Source: CAD feature listing. Evaluate the final solid. Frame: model axes, mm. A direction names the side the tool comes from. Give positions to 0.01 mm unless a question says otherwise; leave off trailing zeros. Order: outer loops, then holes, each group sorted by start corner. A loop starts at its lowest first (then second) coordinate and runs counter-clockwise, first axis right, second up. Notation, with made-up numbers: M -10.5,29.25 L 8.5,29.25 A34 cw 8.5,63.25 Z; hole C -18.5,57.25 d6. An arc over 180 degrees is marked long. Answer as a JSON object with one key per item and string values. Group by question number.
1. Section query B-B (x = 82.45). Output: boundary loops of the cut face in (y, z) (3 decimals).
2. Material intervals for L1, parallel to Z at x = 72.5, y = 22 (3 decimals); L2, parallel to X at y = 53.5, z = 9 (3 decimals); L3, parallel to Z at x = 82.45, y = -2.45 (3 decimals), sorted ascending. Write a range as [from, to].
3. Pull-direction query (X, two-part tool) for faces 1 (the flat face through (143, 11.088, 20)), 2 (the cylindrical face through (135.39, -2.15, 11.51)), 3 (the flat face through (111.252, 40, 102)); classes: +X half, -X half, draft (parallel to the pull), parting line (faces both ways), or undercut.
4. Set-up query: faces 4 (the flat face through (108, 35.1, 92)), 5 (the flat face through (143, 14.753, 52)), 6 (the flat face through (42, 15.306, -3)), 7 (the flat face through (121.69, 32, 69)). Return all of +Z, -Z, +X, -X, +Y, -Y with unobstructed straight access to the full face (end or side cutting, diameter ignored); none if empty.
5. Section query A-A (y = 30). Count the separate pieces of the cut face and the enclosed holes in it, plus the area to 3 significant figures.
6. Pin query (flat end, axial travel): P1, Ø6.5, axis at x = 18.95, z = 12.875, coming from the +Y side; P2, Ø3, axis at y = 54.5, z = 85, coming from the +X side; P3, Ø4, axis at x = 82.45, z = 101.775, coming from the -Y side; P4, Ø0.6, axis at x = 143, y = 16.5, coming from the +Z side. Return the tip coordinate at first contact, or that it passes through.
from build123d import *

# Parameters (mm, degrees)
BOSS_EXTRUDE1_DEPTH = 55.88
SKETCH25_W          = 88.9
SKETCH25_H          = 19.05
CUT_EXTRUDE9_DEPTH  = 45
SKETCH26_W          = 30.523269702
SKETCH26_H          = 2.237493103
SKETCH26_W_2        = 27.906523593
SKETCH26_H_2        = 2.373023229
SKETCH26_W_3        = 27.753916876
SKETCH26_H_3        = 2.119290111
SKETCH26_W_4        = 27.886795766
CUT_EXTRUDE10_DEPTH = 45
SKETCH27_W          = 78.529626093
SKETCH27_H          = 2.934693649
SKETCH27_H_2        = 2.6992147
SKETCH27_H_3        = 2.709324196
CUT_EXTRUDE11_DEPTH = 254
SKETCH23_W          = 12.7
SKETCH23_H          = 12.812800452
CUT_EXTRUDE12_DEPTH = 50.8
SKETCH31_W          = 123.564738067
SKETCH31_H          = 6.504927573
CUT_EXTRUDE13_DEPTH = 113.8
SKETCH34_W          = 2.794
SKETCH34_H          = 6
SKETCH34_W_2        = 3
SKETCH34_H_2        = 6.504927573
CUT_EXTRUDE14_DEPTH = 35.8
SKETCH35_W          = 66.242375008
SKETCH35_H          = 6
CUT_EXTRUDE15_DEPTH = 2.8
BOSS_EXTRUDE2_DEPTH = 3
SKETCH38_W          = 38.1
SKETCH38_H          = 25.4
CUT_EXTRUDE17_DEPTH = 10.16
FILLET1_R           = 2.54
SKETCH37_R          = 2.54
CUT_EXTRUDE18_DEPTH = 5.842
CHAMFER1_SIZE       = 1.27


with BuildPart() as part:
    # Sketch1 → Boss-Extrude1 (new body)
    with BuildSketch(Plane(origin=(0, 0, 0), x_dir=(1, 0, 0), z_dir=(0, 1, 0))):
        Polygon((104.775, 6.175), (-6.175, 6.175), (-6.175, -123.65), (104.902, -123.65), (111.252, -123.65), (111.252, -72.417375008), (145.95, -72.417375008), (145.95, 6.175), align=None)
        Polygon((0, 0), (104.775, 0), (139.775, 0), (139.775, -66.242375008), (107.949403386, -66.242375008), (104.902, -66.242375008), (104.902, -117.475), (0, -117.475), align=None, mode=Mode.SUBTRACT)
    extrude(amount=BOSS_EXTRUDE1_DEPTH)

    # Sketch25 → Cut-Extrude9 (cut)
    with BuildSketch(Plane.ZY.offset(6.175)):
        with Locations((57.39554729, 22.225)):
            Rectangle(SKETCH25_W, SKETCH25_H)
    extrude(amount=-CUT_EXTRUDE9_DEPTH, mode=Mode.SUBTRACT)

    # Sketch26 → Cut-Extrude10 (cut)
    with BuildSketch(Plane(origin=(145.95, 0, 0), x_dir=(0, 0, -1), z_dir=(1, 0, 0))):
        with Locations((-19.859686164, 20.955094684)):
            Rectangle(SKETCH26_W, SKETCH26_H)
        with Locations((-52.150571232, 9.901663162)):
            Rectangle(SKETCH26_W_2, SKETCH26_H_2)
        with Locations((-19.859686164, 9.901663162)):
            Rectangle(SKETCH26_W, SKETCH26_H_2)
        with Locations((-52.074267873, 15.812585987)):
            Rectangle(SKETCH26_W_3, SKETCH26_H_3)
        with Locations((-19.859686164, 15.812585987)):
            Rectangle(SKETCH26_W, SKETCH26_H_3)
        with Locations((-52.140707318, 20.955094684)):
            Rectangle(SKETCH26_W_4, SKETCH26_H)
    extrude(amount=-CUT_EXTRUDE10_DEPTH, mode=Mode.SUBTRACT)

    # Sketch27 → Cut-Extrude11 (cut)
    with BuildSketch(Plane(origin=(0, 0, -6.175), x_dir=(-1, 0, 0), z_dir=(0, 0, -1))):
        with Locations((-41.456138019, 6.407058623)):
            Rectangle(SKETCH27_W, SKETCH27_H)
        with Locations((-41.456138019, 11.590217132)):
            Rectangle(SKETCH27_W, SKETCH27_H_2)
        with Locations((-41.456138019, 16.660698202)):
            Rectangle(SKETCH27_W, SKETCH27_H_3)
    extrude(amount=-CUT_EXTRUDE11_DEPTH, mode=Mode.SUBTRACT)

    # Sketch23 → Cut-Extrude12 (cut)
    with BuildSketch(Plane.XY.offset(72.417375008)):
        with Locations((128.04011729, 32.5625418)):
            Rectangle(SKETCH23_W, SKETCH23_H)
    extrude(amount=-CUT_EXTRUDE12_DEPTH, mode=Mode.SUBTRACT)

    # Sketch31 → Cut-Extrude13 (cut)
    with BuildSketch(Plane.ZY.offset(6.175)):
        with Locations((58.782369034, 48.622896581)):
            Rectangle(SKETCH31_W, SKETCH31_H)
    extrude(amount=-CUT_EXTRUDE13_DEPTH, mode=Mode.SUBTRACT)

    # Sketch34 → Cut-Extrude14 (cut)
    with BuildSketch(Plane.ZY.offset(-107.625)):
        with Locations((67.639375008, 48.370432794)):
            Rectangle(SKETCH34_W, SKETCH34_H)
        with Locations((-1.5, 48.622896581)):
            Rectangle(SKETCH34_W_2, SKETCH34_H_2)
    extrude(amount=-CUT_EXTRUDE14_DEPTH, mode=Mode.SUBTRACT)

    # Sketch35 → Cut-Extrude15 (cut)
    with BuildSketch(Plane.ZY.offset(-139.775)):
        with Locations((33.121187504, 48.370432794)):
            Rectangle(SKETCH35_W, SKETCH35_H)
    extrude(amount=-CUT_EXTRUDE15_DEPTH, mode=Mode.SUBTRACT)

    # Sketch36 → Boss-Extrude2 (add)
    with BuildSketch(Plane.XZ):
        Polygon((111.252, 72.417375008), (111.252, 123.65), (-6.175, 123.65), (-6.175, -6.175), (145.95, -6.175), (145.95, 72.417375008), align=None)
    extrude(amount=BOSS_EXTRUDE2_DEPTH)

    # Sketch38 → Cut-Extrude17 (cut)
    with BuildSketch(Plane(origin=(111.252, 0, 0), x_dir=(0, 0, -1), z_dir=(1, 0, 0))):
        with Locations((-91.9, 22.4)):
            Rectangle(SKETCH38_W, SKETCH38_H)
    extrude(amount=-CUT_EXTRUDE17_DEPTH, mode=Mode.SUBTRACT)

    # Fillet1
    fillet1_edges = [part.edges().sort_by_distance(p)[0] for p in [
        (145.95, 26.44, -6.175),
        (145.95, 26.44, 72.417375008),
        (111.252, 26.44, 123.65),
        (-6.175, 26.44, 123.65),
        (-6.175, 26.44, -6.175),
    ]]
    fillet(fillet1_edges, radius=FILLET1_R)

    # Sketch37 → Cut-Extrude18 (cut)
    with BuildSketch(Plane(origin=(145.95, -3, 72.417375008), x_dir=(1, 0, 0), z_dir=(0, -1, 0))):
        with Locations(Location((-12.7, -59.542375008, 0), (0, 0, 270))):
            Circle(SKETCH37_R)
        with Locations(Location((-63.5, 29.357624992, 0), (0, 0, 270))):
            Circle(SKETCH37_R)
        with Locations(Location((-114.3, 29.357624992, 0), (0, 0, 270))):
            Circle(SKETCH37_R)
        with Locations(Location((-25.4, -59.542375008, 0), (0, 0, 270))):
            Circle(SKETCH37_R)
        with Locations(Location((-38.1, -59.542375008, 0), (0, 0, 270))):
            Circle(SKETCH37_R)
        with Locations(Location((-50.8, -59.542375008, 0), (0, 0, 270))):
            Circle(SKETCH37_R)
        with Locations(Location((-63.5, -59.542375008, 0), (0, 0, 270))):
            Circle(SKETCH37_R)
        with Locations(Location((-76.2, -59.542375008, 0), (0, 0, 270))):
            Circle(SKETCH37_R)
        with Locations(Location((-88.9, -59.542375008, 0), (0, 0, 270))):
            Circle(SKETCH37_R)
        with Locations(Location((-101.6, -59.542375008, 0), (0, 0, 270))):
            Circle(SKETCH37_R)
        with Locations(Location((-114.3, -59.542375008, 0), (0, 0, 270))):
            Circle(SKETCH37_R)
        with Locations(Location((-127, -59.542375008, 0), (0, 0, 270))):
            Circle(SKETCH37_R)
        with Locations(Location((-139.7, -59.542375008, 0), (0, 0, 270))):
            Circle(SKETCH37_R)
    extrude(amount=-CUT_EXTRUDE18_DEPTH, mode=Mode.SUBTRACT)

    # Chamfer1
    chamfer1_edges = [part.edges().sort_by_distance(p)[0] for p in [
        (133.25, 0, 15.415),
        (6.25, 0, 15.415),
        (18.95, 0, 15.415),
        (31.65, 0, 15.415),
        (44.35, 0, 15.415),
        (82.45, 0, 104.315),
        (31.65, 0, 104.315),
        (120.55, 0, 15.415),
        (107.85, 0, 15.415),
        (95.15, 0, 15.415),
        (82.45, 0, 15.415),
        (69.75, 0, 15.415),
        (57.05, 0, 15.415),
    ]]
    chamfer(chamfer1_edges, length=CHAMFER1_SIZE)


solid = part.part
Answer sheet:
{
 "1": {"outline": "M -3,-6.175 L 55.88,-6.175 L 55.88,0 L 51.875,0 L 51.875,-3 L 45.37,-3 L 45.37,0 L 0,0 L 0,9.065 L -1.27,10.335 L -3,10.335 Z; M -3,15.415 L -1.27,15.415 L 0,16.685 L 0,97.965 L -1.27,99.235 L -3,99.235 Z; M -3,104.315 L -1.27,104.315 L 0,105.585 L 0,117.475 L 45.37,117.475 L 45.37,120.565 L 51.875,120.565 L 51.875,117.475 L 55.88,117.475 L 55.88,123.65 L -3,123.65 Z"},
 "2": {"L1": "[-6.175, 0], [117.475, 123.65]", "L2": "[-6.175, 0], [139.775, 145.95]", "L3": "[-6.175, 10.335], [15.415, 99.235], [104.315, 123.65]"},
 "3": {"face 1": "draft", "face 2": "undercut", "face 3": "+X half"},
 "4": {"face 4": "+X", "face 5": "+X, -X", "face 6": "+Z, -Z", "face 7": "+Z"},
 "5": {"separate pieces": "3", "enclosed holes": "0", "area": "2,460 mm^2"},
 "6": {"P1": "y = -0.56", "P2": "x = 111.25", "P3": "through", "P4": "z = 72.42"}
}
